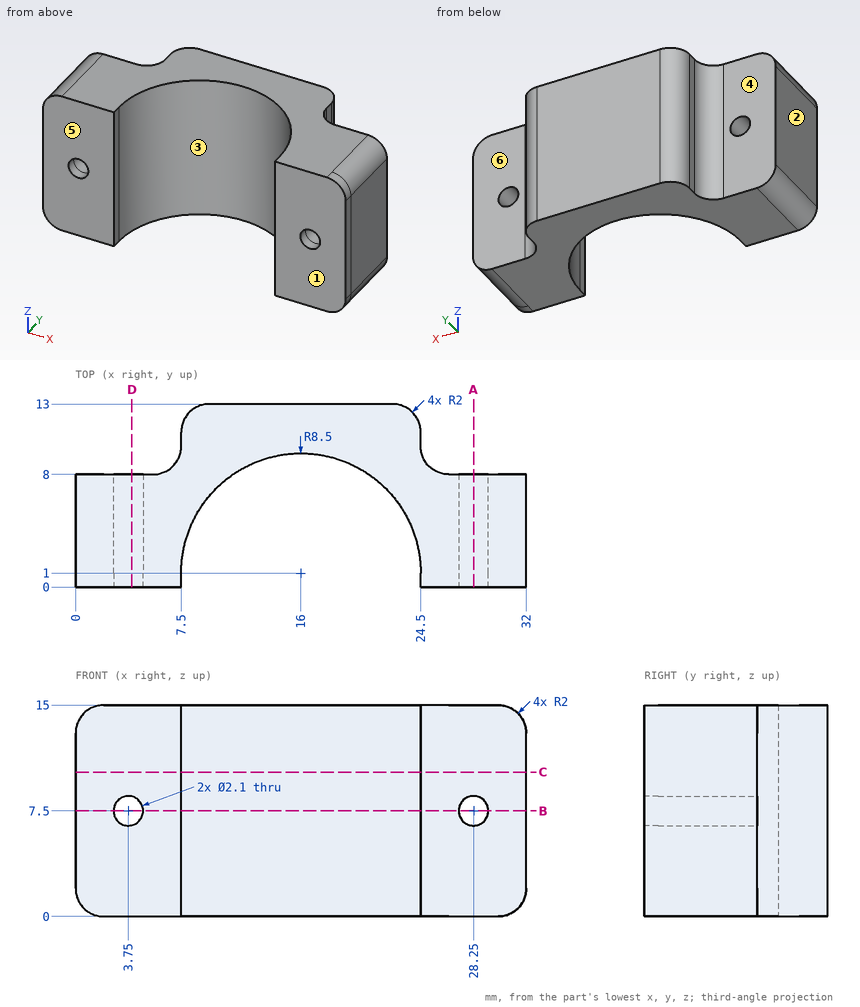
Check sheet for the drawn part. Datum: minimum x, y, z corner. Units: mm. A direction names the side the tool comes from. Round coordinates to 2 decimals unless told otherwise and drop trailing zeros. Loops run counter-clockwise (first coordinate to the right, second up) from the corner with the lowest first, then second, coordinate; pieces in that order, holes last. Notation, with made-up numbers: (69.5, 13) - (116.5, 13) arc R18 cw to (116.5, 21) - close; hole circle Ø11 at (-21.5, 52.5). An arc over 180 degrees is marked (long way). Write each question's results on one line, items separated by ' | '. Start each with the question number.
Q1. Access from +Z, -Z, +X, -X, +Y, -Y to the whole of each face (thin tool, end or side, straight path). Record for the marked faces 4, 5 and 6.
Q2. Cross-section at A-A on x = 28.25. Enter the section's corners in (y, z).
Q3. Cross-section at C-C on z = 10.25. Enter the section's corners in (x, y).
Q4. Release check for a two-part mould opening along X. For the marked faces 1, 2 and 3 record: +X half, -X half, draft (parallel to the pull), parting line (faces both ways), or undercut.
Q5. Cross-section at B-B on z = 7.5. Enter the section's corners in (x, y), and give its area (3 significant figures).
Q6. Gauge pin test, flat ends, axial feed: P1, Ø3, axis at x = 4, z = 8.5, coming from the +Y side; P2, Ø1.1, axis at y = 10.5, z = 7, coming from the -X side; P3, Ø0.8, axis at y = 10.5, z = 4.5, coming from the +X side. Record the tip position at first contact, or that the pin passes through.
Q7. Cross-section at D-D on x = 4. Enter the section's corners in (y, z), and give its area (3 significant figures).
Q8. Thickness scan on line 1 (X direction, y = 0.7, z = 7.5); line 2 (Z direction, x = 3.75, y = 0.7); line 3 (X direction, y = 2.75, z = 7.5). Record the ranges inside material, lowest first. Write a range as [from, to].
Answers below:
1) face 4: +Z, -Z, -X, +Y | face 5: +Z, -Z, +X, -X, -Y | face 6: +Z, -Z, +X, +Y
2) outline: (0, 0) - (8, 0) - (8, 6.45) - (0, 6.45) - close; (0, 8.55) - (8, 8.55) - (8, 15) - (0, 15) - close
3) outline: (0, 0) - (7.5, 0) - (7.5, 1) arc R8.5 cw to (24.5, 1) - (24.5, 0) - (32, 0) - (32, 8) - (26.5, 8) arc R2 cw to (24.5, 10) - (24.5, 11) arc R2 ccw to (22.5, 13) - (9.5, 13) arc R2 ccw to (7.5, 11) - (7.5, 10) arc R2 cw to (5.5, 8) - (0, 8) - close
4) face 1: draft | face 2: -X half | face 3: undercut
5) outline: (0, 0) - (2.7, 0) - (2.7, 8) - (0, 8) - close; (4.8, 0) - (7.5, 0) - (7.5, 1) arc R8.5 cw to (24.5, 1) - (24.5, 0) - (27.2, 0) - (27.2, 8) - (26.5, 8) arc R2 cw to (24.5, 10) - (24.5, 11) arc R2 ccw to (22.5, 13) - (9.5, 13) arc R2 ccw to (7.5, 11) - (7.5, 10) arc R2 cw to (5.5, 8) - (4.8, 8) - close; (29.3, 0) - (32, 0) - (32, 8) - (29.3, 8) - close | area: 177 mm²
6) P1: stops at y = 8 | P2: stops at x = 7.5 | P3: stops at x = 24.5
7) outline: (0, 0) - (8, 0) - (8, 6.48) - (0, 6.48) - close; (0, 8.52) - (8, 8.52) - (8, 15) - (0, 15) - close | area: 104 mm²
8) line 1: x = [0, 2.7], [4.8, 7.5], [24.5, 27.2], [29.3, 32] | line 2: z = [0, 6.45], [8.55, 15] | line 3: x = [0, 2.7], [4.8, 7.68], [24.32, 27.2], [29.3, 32]
